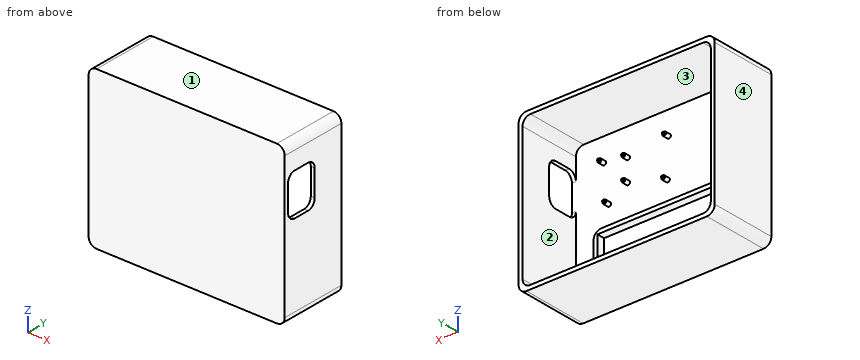
from build123d import *

# Parameters (mm, degrees)
SKETCH2_W           = 250
SKETCH2_H           = 200
BOSS_EXTRUDE1_DEPTH = 5
SKETCH3_W           = 250
SKETCH3_H           = 200
SKETCH3_W_2         = 240
SKETCH3_H_2         = 190
BOSS_EXTRUDE2_DEPTH = 80
SKETCH1_W           = 178
SKETCH1_H           = 68
SKETCH1_W_2         = 168
SKETCH1_H_2         = 58
BOSS_EXTRUDE3_DEPTH = 10
SKETCH7_R           = 2.5
BOSS_EXTRUDE4_DEPTH = 7
SKETCH8_R           = 1.4
BOSS_EXTRUDE5_DEPTH = 2
CUT_EXTRUDE1_REACH  = 284.356
SKETCH4_W           = 53.3
SKETCH4_H           = 40
FILLET1_R           = 10


with BuildPart() as part:
    # Sketch2 → Boss-Extrude1 (new body)
    with BuildSketch(Plane(origin=(0, 0, 0), x_dir=(1, 0, 0), z_dir=(0, 1, 0))):
        Rectangle(SKETCH2_W, SKETCH2_H)
    extrude(amount=BOSS_EXTRUDE1_DEPTH)

    # Sketch3 → Boss-Extrude2 (add)
    with BuildSketch(Plane(origin=(0, 5, 0), x_dir=(1, 0, 0), z_dir=(0, 1, 0))):
        Rectangle(SKETCH3_W, SKETCH3_H)
        Rectangle(SKETCH3_W_2, SKETCH3_H_2, mode=Mode.SUBTRACT)
    extrude(amount=BOSS_EXTRUDE2_DEPTH)

    # Sketch1 → Boss-Extrude3 (add)
    with BuildSketch(Plane(origin=(0, 5, 0), x_dir=(1, 0, 0), z_dir=(0, 1, 0))):
        with Locations((0, 47.5)):
            Rectangle(SKETCH1_W, SKETCH1_H)
        with Locations((0, 47.5)):
            Rectangle(SKETCH1_W_2, SKETCH1_H_2, mode=Mode.SUBTRACT)
    extrude(amount=BOSS_EXTRUDE3_DEPTH)

    # Sketch7 → Boss-Extrude4 (add)
    with BuildSketch(Plane(origin=(0, 5, 0), x_dir=(1, 0, 0), z_dir=(0, 1, 0))):
        with Locations(Location((2.7, -16.7, 0), (0, 0, 90))):
            Circle(SKETCH7_R)
        with Locations(Location((1.4, -64.9, 0), (0, 0, 90))):
            Circle(SKETCH7_R)
        with Locations(Location((53.5, -31.9, 0), (0, 0, 90))):
            Circle(SKETCH7_R)
        with Locations(Location((77.6, -16.7, 0), (0, 0, 90))):
            Circle(SKETCH7_R)
        with Locations(Location((83.95, -64.9, 0), (0, 0, 90))):
            Circle(SKETCH7_R)
        with Locations(Location((53.5, -59.8, 0), (0, 0, 90))):
            Circle(SKETCH7_R)
    extrude(amount=BOSS_EXTRUDE4_DEPTH)

    # Sketch8 → Boss-Extrude5 (add)
    with BuildSketch(Plane(origin=(0, 12, 0), x_dir=(1, 0, 0), z_dir=(0, 1, 0))):
        with Locations(Location((2.7, -16.7, 0), (0, 0, 270))):
            Circle(SKETCH8_R)
        with Locations(Location((53.5, -31.9, 0), (0, 0, 270))):
            Circle(SKETCH8_R)
        with Locations(Location((77.6, -16.7, 0), (0, 0, 270))):
            Circle(SKETCH8_R)
        with Locations(Location((53.5, -59.8, 0), (0, 0, 270))):
            Circle(SKETCH8_R)
        with Locations(Location((1.4, -64.9, 0), (0, 0, 270))):
            Circle(SKETCH8_R)
        with Locations(Location((83.95, -64.9, 0), (0, 0, 270))):
            Circle(SKETCH8_R)
    extrude(amount=BOSS_EXTRUDE5_DEPTH)

    # Sketch4 → Cut-Extrude1 (cut, up to next)
    with BuildSketch(Plane(origin=(125, 0, 0), x_dir=(0, 0, -1), z_dir=(1, 0, 0)), mode=Mode.PRIVATE) as cut_extrude1_sk1:
        with Locations((-40.75, 25)):
            Rectangle(SKETCH4_W, SKETCH4_H)
    cut_extrude1_tool1 = extrude(cut_extrude1_sk1.sketch, amount=-CUT_EXTRUDE1_REACH, mode=Mode.PRIVATE) & part.part
    add(cut_extrude1_tool1.solids().sort_by_distance((125, 25, 40.75))[0], mode=Mode.SUBTRACT)

    # Fillet1
    fillet1_edges = [part.edges().sort_by_distance(p)[0] for p in [
        (122.5, 5, 67.4),
        (122.5, 45, 67.4),
        (122.5, 45, 14.1),
        (122.5, 5, 14.1),
        (120, 45, 95),
        (120, 45, -95),
        (-120, 45, -95),
        (-120, 45, 95),
        (-89, 10, -13.5),
        (89, 10, -13.5),
        (89, 10, -81.5),
        (-89, 10, -81.5),
        (125, 42.5, 100),
        (-125, 42.5, 100),
        (-125, 42.5, -100),
        (125, 42.5, -100),
    ]]
    fillet(fillet1_edges, radius=FILLET1_R)


solid = part.part
Model file for the job. Use its own axes, mm. Face numbers are marked on the shaded views. Coordinates: 2 decimals unless noted, no trailing zeros. Order: outer loops, then holes, each group sorted by start corner. A loop starts at its lowest first (then second) coordinate and runs counter-clockwise, first axis right, second up. Notation, with made-up numbers: M 15.5,84 L 24.5,84 A10 cw 24.5,89 Z; hole C 76.25,-12 d9. An arc over 180 degrees is marked long. Return JSON: item names as keys, results as strings.
1. Saw through at A-A (z = 43). Give the cut face in (x, y).
Ans:
{"outline": "M -125,0 L 125,0 L 125,5 L -120,5 L -120,85 L -125,85 Z; M 120,45 L 125,45 L 125,85 L 120,85 Z"}
2. Flat gauge pins, fed straight in: pin 1 (2 mm diameter, centred on x = 17, z = -52, fed in from +Y); pin 2 (4 mm diameter, centred on x = 7, z = -18.5, fed in from +Y); pin 3 (4 mm diameter, centred on x = 123, y = 21, fed in from +Z). Where does each tip first touch, or does it go through?
Ans:
{"pin 1": "y = 5", "pin 2": "y = 15", "pin 3": "z = 98"}
3. Saw through at D-D (z = -53). Give the cut face in (x, y), and give its area (3 significant figures).
Ans:
{"outline": "M -125,0 L 125,0 L 125,85 L 120,85 L 120,5 L 89,5 L 89,15 L 84,15 L 84,5 L -84,5 L -84,15 L -89,15 L -89,5 L -120,5 L -120,85 L -125,85 Z", "area": "2,150 mm^2"}
4. Drill centre lines: probe 1 along Z at (x, y) = (5, 21); probe 2 along X at (y, z) = (62.5, -33.5); probe 3 along Y at (x, z) = (-29, 22). Where is each one in solid material? Low to high.
Ans:
{"probe 1": "-100 to -95, 95 to 100", "probe 2": "-125 to -120, 120 to 125", "probe 3": "0 to 5"}
5. Saw through at C-C (x = 34). Give the cut face in (y, z).
Ans:
{"outline": "M 0,-100 L 85,-100 L 85,-95 L 5,-95 L 5,-81.5 L 15,-81.5 L 15,-76.5 L 5,-76.5 L 5,-18.5 L 15,-18.5 L 15,-13.5 L 5,-13.5 L 5,95 L 85,95 L 85,100 L 0,100 Z"}
6. Saw through at B-B (y = 48). Give the cut face in (x, z), and give its area (3 significant figures).
Ans:
{"outline": "M -125,-90 A10 ccw -115,-100 L 115,-100 A10 ccw 125,-90 L 125,90 A10 ccw 115,100 L -115,100 A10 ccw -125,90 Z; hole M -120,-85 A10 ccw -110,-95 L 110,-95 A10 ccw 120,-85 L 120,85 A10 ccw 110,95 L -110,95 A10 ccw -120,85 Z", "area": "4,400 mm^2"}
7. Pull direction X, two halves, no side cores. Call the marked faces 1, 2, 3 and 4: +X half, -X half, draft (parallel to the pull), parting line (faces both ways), or undercut.
Ans:
{"face 1": "draft", "face 2": "undercut", "face 3": "undercut", "face 4": "-X half"}
